The drawing under review shows one solid part. Ordinate dimensions are in mm from its lowest x, y, z. A direction names the side the tool comes from. Give positions to 0.01 mm unless a question says otherwise; leave off trailing zeros. Order: outer loops, then holes, each group sorted by start corner. A loop starts at its lowest first (then second) coordinate and runs counter-clockwise, first axis right, second up. Notation, with made-up numbers: (-11.5, 77) -> (14.5, 77) arc R33 ccw to (14.5, 109) -> close; hole circle Ø7 at (9.5, 38.25). An arc over 180 degrees is marked (long way). One line per item, written item: value. Start each with the question number.
1) Consider section D-D (y = 63.5). State the section outline as (x, z) points (3 decimals), plus the area to 3 significant figures.
2) Wall thickness on line 1 along Y through (x, z) = (44.45, 8.25); line 2 along Y through (x, z) = (44.45, 2.5); line 3 along Z through (x, y) = (19.5, 15.5): over which ranges is each line inside the solid? List them lowest first. Write a range as from..to.
3) Tool access review of the marked faces 1 and 2: name each direction out of +Z, -Z, +X, -X, +Y, -Y from which nothing blocks a thin tool from reaching the whole face with its end or side.
4) For pin 1 (2 mm diameter, centred on y = 71.5, z = 10, fed in from -X); pin 2 (3 mm diameter, centred on x = 73, z = 5, fed in from -Y); pin 3 (1.5 mm diameter, centred on y = 47.5, z = 2, fed in from +X), all flat-tipped, find the tip position at first contact; note any pin that passes through.
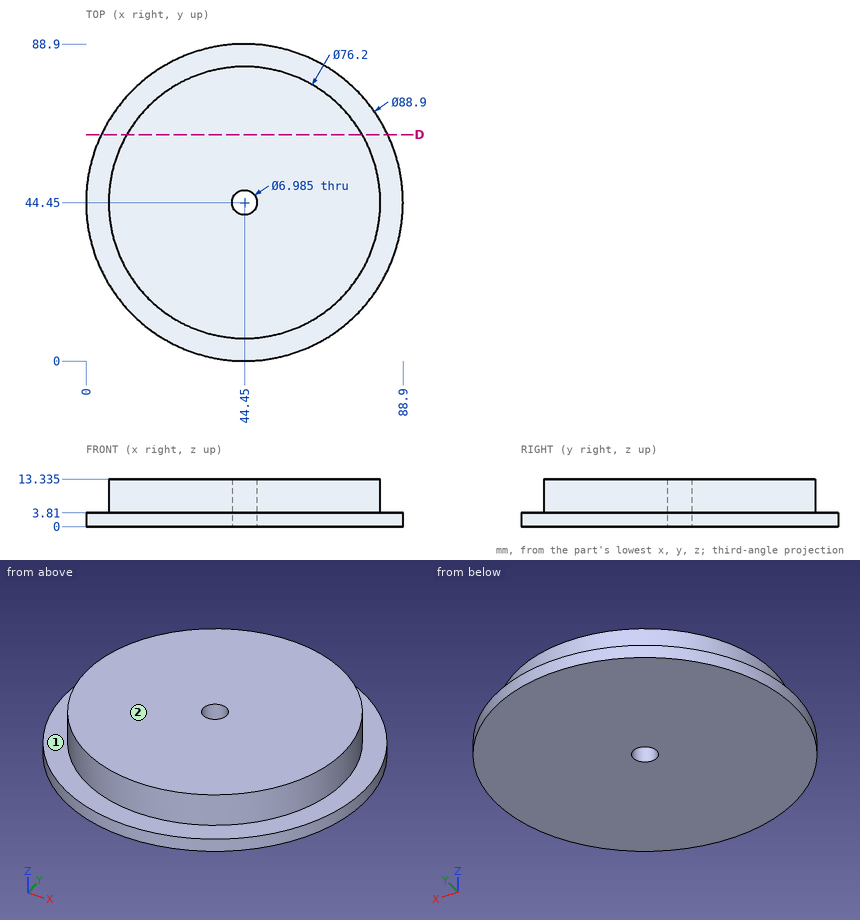
Checked values:
1. outline: (4.289, 0) -> (84.611, 0) -> (84.611, 3.81) -> (77.446, 3.81) -> (77.446, 13.335) -> (11.454, 13.335) -> (11.454, 3.81) -> (4.289, 3.81) -> close
1. area: 935 mm^2
2. line 1: y = 6.35..40.96, 47.94..82.55
2. line 2: y = 0..40.96, 47.94..88.9
2. line 3: z = 0..3.81
3. face 1: +Z
3. face 2: +Z, +X, -X, +Y, -Y
4. pin 1: stops at x = 16.65
4. pin 2: stops at y = 9.64
4. pin 3: stops at x = 88.84
